Autodesk Inventor part; units mm, degrees
ref_plane "YZ Plane" through (0, 0, 0) normal (1, 0, 0) x (0, 1, 0)
ref_plane "XZ Plane" through (0, 0, 0) normal (0, 1, 0) x (-1, 0, 0)
ref_plane "XY Plane" through (0, 0, 0) normal (0, 0, 1) x (1, 0, 0)
sketch "Esquisse1" plane through (0, 0, 0) normal (1, 0, 0) x (0, 1, 0)
  line L0 (15, 8.5) -> (-15, 8.5)
  line L1 (-15, 8.5) -> (-15, -8.5)
  line L2 (-15, -8.5) -> (15, -8.5)
  line L3 (15, -8.5) -> (15, 8.5)
  point P0 (0, 0)
  point P1 (0, 0)
  point P2 (0, 0)
  dimension "d4" = 30
  dimension "d5" = 17
extrude "Extrusion1" add sketch "Esquisse1" along normal blind 10
sketch "Esquisse2" plane through (10, 0, 0) normal (1, 0, 0) x (0, 0, -1)
  line L0 (-7.5, 13.5) -> (7.5, 13.5)
  line L1 (7.5, 13.5) -> (7.5, -13.5)
  line L2 (7.5, -13.5) -> (-7.5, -13.5)
  line L3 (-7.5, -13.5) -> (-7.5, 13.5)
  line L4 (-7.5, 13.5) -> (7.5, -13.5)
  line L5 (-7.5, -13.5) -> (7.5, 13.5)
  point P0 (0, 0)
  point P1 (0, 0)
  point P2 (0, 0)
  dimension "d8" = 27
  dimension "d9" = 15
extrude "Extrusion2" cut sketch "Esquisse2" against normal blind 9
sketch "Esquisse3" plane through (1, 0, 0) normal (1, 0, 0) x (0, 0, -1)
  line L0 (7.5, -13.5) -> (-7.5, -13.5)
  line L1 (7.5, 13.5) -> (7.5, -13.5)
  line L2 (-7.5, -13.5) -> (7.5, -13.5)
  line L3 (7.5, -13.5) -> (7.5, -7.5)
  line L4 (7.5, -7.5) -> (-7.5, -7.5)
  line L5 (-7.5, -7.5) -> (-7.5, -13.5)
  point P0 (0, 0)
  dimension "d12" = 6
extrude "Extrusion3" cut sketch "Esquisse3" against normal blind 9
properties part number "support_tof_actionneur_panneaux_solaires"
Build history of the part. All positions in model axes, mm. A direction names the side the tool comes from. Coordinates: 2 decimals unless noted, no trailing zeros. Write each loop counter-clockwise with the first axis right and the second up, starting at its lowest first coordinate (ties: lowest second). Pieces come first, ordered by that corner, then holes.
1. Drop a flat-ended pin along its axis: pin 1 (6 mm diameter, centred on y = -9.5, z = 4, fed in from +X). Give the stop position or say it passes through.
Answer block:
pin 1: stops at x = 1
2. Band-saw the part on B-B, the plane y = -10.5. Give the cut face in (x, z), and give its area (3 significant figures).
Answer block:
outline: (0, -8.5) - (10, -8.5) - (10, -7.5) - (0, -7.5) - close; (0, 7.5) - (10, 7.5) - (10, 8.5) - (0, 8.5) - close
area: 20.0 mm2
3. Drill centre lines: probe 1 along Y at (x, z) = (7.5, -0.5); probe 2 along Z at (x, y) = (4.5, -5.5); probe 3 along Y at (x, z) = (0.75, 0.75). Where is each one in solid material? Low to high.
Answer block:
probe 1: y = -15 to -13.5, 13.5 to 15
probe 2: z = -8.5 to -7.5, 7.5 to 8.5
probe 3: y = -15 to -13.5, -7.5 to 15
4. Band-saw the part on C-C, the plane x = 5.5. Give the cut face in (y, z), and give its area (3 significant figures).
Answer block:
outline: (-15, -8.5) - (15, -8.5) - (15, 8.5) - (-15, 8.5) - close; hole (-13.5, -7.5) - (13.5, -7.5) - (13.5, 7.5) - (-13.5, 7.5) - close
area: 105 mm2
5. Pull direction Y, two halves, no side cores. Call faces 1 (the flat face through (5, -15, 0)), 2 (the flat face through (5, 15, 0)), 3 (the flat face through (0, 0, 0)), 4 (the flat face through (5, -13.5, 0)): released by +Y, released by -Y, zero draft, split by the parting line, or undercut.
Answer block:
face 1: released by -Y
face 2: released by +Y
face 3: zero draft
face 4: undercut
6. Band-saw the part on D-D, the plane y = 12.5. Give the cut face in (x, z), and give its area (3 significant figures).
Answer block:
outline: (0, -8.5) - (10, -8.5) - (10, -7.5) - (1, -7.5) - (1, 7.5) - (10, 7.5) - (10, 8.5) - (0, 8.5) - close
area: 35.0 mm2
7. 3-axis set-ups, long thin cutter, end or side, ignore diameter. For faces 5 (the flat face through (5, 0, 8.5)), 6 (the flat face through (0.5, -7.5, -0.1)), 7 (the flat face through (1, 3, 0)): which of +Z, -Z, +X, -X, +Y, -Y reach the whole face in a straight line?
Answer block:
face 5: +Z, +X, -X, +Y, -Y
face 6: +X, -X
face 7: +X
8. Band-saw the part on A-A, the plane z = -5.5. Give the cut face in (x, y), and give its area (3 significant figures).
Answer block:
outline: (0, -15) - (10, -15) - (10, -13.5) - (0, -13.5) - close; (0, -7.5) - (1, -7.5) - (1, 13.5) - (10, 13.5) - (10, 15) - (0, 15) - close
area: 51.0 mm2
